```python
from build123d import *

# Parameters (mm, degrees)
RESSALTO_EXTRUS_O1_DEPTH = 79
RESSALTO_EXTRUS_O2_DEPTH = 1
ESBO_O4_W                = 23.972124634
ESBO_O4_H                = 25
CORTE_EXTRUS_O1_DEPTH    = 80.807757613


with BuildPart() as part:
    # Esboço1 → Ressalto-extrusão1 (new, symmetric)
    with BuildSketch(Plane.XY):
        Polygon((-3, 0), (3, 0), (6.061467459, 7.39103626), (7.262510851, 6.893547798), (3.868632229, -1.3), (-3.868632229, -1.3), (-7.262510851, 6.893547798), (-6.061467459, 7.39103626), align=None)
    extrude(amount=RESSALTO_EXTRUS_O1_DEPTH, both=True)

    # Esboço2 → Ressalto-extrusão2 (add)
    with BuildSketch(Plane(origin=(0, 0, -79), x_dir=(-1, 0, 0), z_dir=(0, 0, -1))):
        Polygon((-6.061467459, 7.39103626), (6.061467459, 7.39103626), (7.262510851, 6.893547798), (3.868632229, -1.3), (-3.868632229, -1.3), (-7.262510851, 6.893547798), align=None)
    ressalto_extrus_o2 = extrude(amount=-RESSALTO_EXTRUS_O2_DEPTH)

    # Espelhar1: Ressalto-extrusão2 across plane
    add(ressalto_extrus_o2.mirror(Plane.XY))

    # Esboço4 → Corte-extrusão1 (cut, through all)
    with BuildSketch(Plane.XZ.offset(1.3)):
        with Locations((8.986062317, 0)):
            Rectangle(ESBO_O4_W, ESBO_O4_H)
    extrude(amount=-CORTE_EXTRUS_O1_DEPTH, mode=Mode.SUBTRACT)


solid = part.part
```
Work out the finished part from the listing and answer in its coordinate system (mm). A direction names the side the tool comes from. Give positions to 0.01 mm unless a question says otherwise; leave off trailing zeros. Write each loop counter-clockwise with the first axis right and the second up, starting at its lowest first coordinate (ties: lowest second). Pieces come first, ordered by that corner, then holes. Notation, with made-up numbers: (0, -6.75) - (23, -6.75) arc R26 ccw to (23, 10.25) - close; hole circle Ø1 at (33.5, -37.75). An arc over 180 degrees is marked (long way). Use one line per item in the form item = value.
1. Consider L1, parallel to Z at x = 5.5, y = 3.25; L2, parallel to Z at x = -3, y = 0.75; L3, parallel to Y at x = 0, z = 36.5. Determine where each line is inside the solid, lowest interval first.
Filled in:
L1 = -79 to -12.5, 12.5 to 79
L2 = -79 to -78, 78 to 79
L3 = -1.3 to 0
2. A cutting plane is placed at D-D (z = 8). Write down the section's boundary in (x, y).
Filled in:
outline = (-7.26, 6.89) - (-3.87, -1.3) - (-3, -1.3) - (-3, 0) - (-6.06, 7.39) - close
3. For faces 1 (the face through (4, 1, -12.5)), 2 (the face through (0, 4, 79)), 3 (the face through (0, 0, -45)), determine the directions among +Z, -Z, +X, -X, +Y, -Y from which every point of the face is accessible in a straight line to the end or side of a thin tool.
Filled in:
face_1 = +X, +Y, -Y
face_2 = +Z, +X, -X, +Y, -Y
face_3 = +Y
4. A cutting plane is placed at B-B (z = -27). Write down the section's boundary in (x, y).
Filled in:
outline = (-7.26, 6.89) - (-3.87, -1.3) - (3.87, -1.3) - (7.26, 6.89) - (6.06, 7.39) - (3, 0) - (-3, 0) - (-6.06, 7.39) - close
5. A cutting plane is placed at A-A (x = -1.5). Write down the section's boundary in (y, z), and give its area (3 significant figures).
Filled in:
outline = (-1.3, -79) - (7.39, -79) - (7.39, -78) - (0, -78) - (0, -12.5) - (-1.3, -12.5) - close; (-1.3, 12.5) - (0, 12.5) - (0, 78) - (7.39, 78) - (7.39, 79) - (-1.3, 79) - close
area = 188 mm^2
6. Each of these flat-tipped pins is pushed along its axis until it touches: pin 1 Ø6 at (x, z) = (-0.5, 5.5) entering from +Y; pin 2 Ø1.5 at (x, z) = (-4, 15) entering from +Y; pin 3 Ø1.8 at (x, z) = (-1, -42) entering from +Y. Where does it stop, or does it pass through?
Filled in:
pin_1 = 1.21
pin_2 = 4.22
pin_3 = 0
7. A cutting plane is placed at C-C (y = 5). Write down the section's boundary in (x, z).
Filled in:
outline = (-6.48, -79) - (6.48, -79) - (6.48, -12.5) - (5.07, -12.5) - (5.07, -78) - (-5.07, -78) - (-5.07, 78) - (5.07, 78) - (5.07, 12.5) - (6.48, 12.5) - (6.48, 79) - (-6.48, 79) - close
8. Determine the mould class of faces 4 (the face through (0, 4, -79)), 5 (the face through (0, 0, 46)), 6 (the face through (-5.54, 2.74, 1.11)), 7 (the face through (-4.552, 3.747, 1.092)) for opening direction Z: released by +Z, released by -Z, zero draft, split by the parting line, or undercut.
Filled in:
face_4 = released by -Z
face_5 = undercut
face_6 = zero draft
face_7 = undercut
